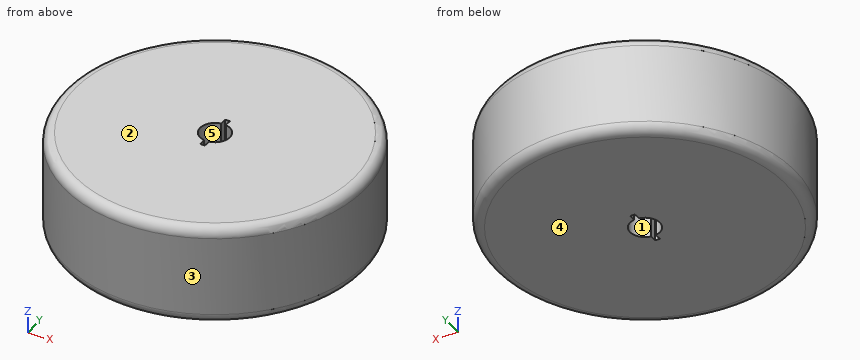
from build123d import *

# Parameters (mm, degrees)
SKETCH1_R           = 38.1
BOSS_EXTRUDE1_DEPTH = 25.4
CUT_EXTRUDE1_REACH  = 61.568
SKETCH2_R           = 3.81
FILLET1_R           = 2.54
FILLET2_R           = 2.54
CUT_EXTRUDE2_START  = -25.4
SKETCH3_W           = 1.220415144
SKETCH3_H           = 11.022652864
CUT_EXTRUDE2_DEPTH  = 25.4


with BuildPart() as part:
    # Sketch1 → Boss-Extrude1 (new body)
    with BuildSketch(Plane.XY):
        Circle(SKETCH1_R)
    extrude(amount=BOSS_EXTRUDE1_DEPTH)

    # Sketch2 → Cut-Extrude1 (cut, up to next)
    with BuildSketch(Plane.XY.offset(25.4), mode=Mode.PRIVATE) as cut_extrude1_sk1:
        Circle(SKETCH2_R)
    cut_extrude1_tool1 = extrude(cut_extrude1_sk1.sketch, amount=-CUT_EXTRUDE1_REACH, mode=Mode.PRIVATE) & part.part
    add(cut_extrude1_tool1.solids().sort_by_distance((0, 0, 25.4))[0], mode=Mode.SUBTRACT)

    # Fillet1
    fillet1_edges = [part.edges().sort_by_distance(p)[0] for p in [
        (-38.1, 0, 25.4),
    ]]
    fillet(fillet1_edges, radius=FILLET1_R)

    # Fillet2
    fillet2_edges = [part.edges().sort_by_distance(p)[0] for p in [
        (-38.1, 0, 0),
    ]]
    fillet(fillet2_edges, radius=FILLET2_R)

    # Sketch3 → Cut-Extrude2 (cut)
    with BuildSketch(Plane.XY.offset(25.4).offset(CUT_EXTRUDE2_START)):
        Rectangle(SKETCH3_W, SKETCH3_H)
    extrude(amount=CUT_EXTRUDE2_DEPTH, mode=Mode.SUBTRACT)


solid = part.part
Check sheet for the modelled part. Datum: model origin and axes. Units: mm. Face numbers are marked on the shaded views. A direction names the side the tool comes from. Give positions to 0.01 mm unless a question says otherwise; leave off trailing zeros. Write each loop counter-clockwise with the first axis right and the second up, starting at its lowest first coordinate (ties: lowest second). Pieces come first, ordered by that corner, then holes. Notation, with made-up numbers: (49, -3.5) -> (92, -3.5) arc R8 cw to (92, 3.5) -> close; hole circle Ø7 at (51.5, 38.25). An arc over 180 degrees is marked (long way). One line per item, written item: value. Start each with the question number.
Item 1: Draft check along X on the marked faces 3, 4 and 5. Enter one of: +X half, -X half, draft (parallel to the pull), parting line (faces both ways), or undercut.
Item 2: Section check B-B on z = 4. Record the cut outline in (x, y), then the cut area to 3 significant figures.
Item 3: Section check A-A on y = 0. Record the cut outline in (x, z).
Item 4: Material ranges on probe 1 along X at (y, z) = (-0.5, 2.5); probe 2 along X at (y, z) = (2, 21.5); probe 3 along Y at (x, z) = (-2.5, 5.75), recorded low to high. Write a range as from..to.
Item 5: Tool access check on the marked faces 1 and 2. Record the directions out of +Z, -Z, +X, -X, +Y, -Y that give a thin tool (end or side, any length) a straight path to the whole face; none if there is none.
Item 6: Gauge pin test, flat ends, axial feed: pin 1 (12 mm diameter, centred on x = -13, z = 13.5, fed in from -Y); pin 2 (4 mm diameter, centred on x = 4, z = 21.5, fed in from +Y); pin 3 (1.4 mm diameter, centred on y = -4.5, z = 15.5, fed in from -X). Record the tip position at first contact, or that the pin passes through.
Results list:
1. face 3: parting line
1. face 4: draft
1. face 5: undercut
2. outline: circle Ø76.2 at (0, 0); hole (-0.61, -5.51) -> (0.61, -5.51) -> (0.61, -3.76) arc R3.81 ccw to (0.61, 3.76) -> (0.61, 5.51) -> (-0.61, 5.51) -> (-0.61, 3.76) arc R3.81 ccw to (-0.61, -3.76) -> close
2. area: 4,510 mm²
3. outline: (-38.1, 2.54) arc R2.54 ccw to (-35.56, 0) -> (-3.81, 0) -> (-3.81, 25.4) -> (-35.56, 25.4) arc R2.54 ccw to (-38.1, 22.86) -> close; (3.81, 0) -> (35.56, 0) arc R2.54 ccw to (38.1, 2.54) -> (38.1, 22.86) arc R2.54 ccw to (35.56, 25.4) -> (3.81, 25.4) -> close
4. probe 1: -38.1..-3.78, 3.78..38.1
4. probe 2: -38.05..-3.24, 3.24..38.05
4. probe 3: -38.02..-2.88, 2.88..38.02
5. face 1: +Z, -Z
5. face 2: +Z, +X, -X, +Y, -Y
6. pin 1: y = -37.45
6. pin 2: y = 38.05
6. pin 3: x = -37.91
